```python
from build123d import *

# Parameters (mm, degrees)
SKETCH1_R           = 0.3
SKETCH1_W           = 2
SKETCH1_H           = 1.5
BOSS_EXTRUDE1_DEPTH = 1.7272


with BuildPart() as part:
    # Sketch1 → Boss-Extrude1 (new body)
    # profile 1 of 3: a face of its own
    with BuildSketch(Plane(origin=(0, 0, 0), x_dir=(0, 0, -1), z_dir=(1, 0, 0))):
        with BuildLine():
            ThreePointArc((-0.95, 14.390683939), (0, 15.340683939), (0.95, 14.390683939))
            Line((0.95, 14.390683939), (0.95, 12.490683939))
            Line((0.95, 12.490683939), (2.5, 12.490683939))
            Line((2.5, 12.490683939), (2.5, 4.605171007))
            ThreePointArc((2.5, 4.605171007), (5.185747801, 0.752076956), (3.705239533, -3.705239533))
            Line((3.705239533, -3.705239533), (2.644579362, -2.644579362))
            ThreePointArc((2.644579362, -2.644579362), (0, 3.74), (-2.644579362, -2.644579362))
            Line((-2.644579362, -2.644579362), (-3.705239533, -3.705239533))
            ThreePointArc((-3.705239533, -3.705239533), (-5.185747801, 0.752076956), (-2.5, 4.605171007))
            Line((-2.5, 4.605171007), (-2.5, 12.490683939))
            Line((-2.5, 12.490683939), (-0.95, 12.490683939))
            Line((-0.95, 12.490683939), (-0.95, 14.390683939))
        make_face()
        with Locations((0, 14.690683939)):
            Circle(SKETCH1_R, mode=Mode.SUBTRACT)
    # profile 2 of 3: a face of its own
    with BuildSketch(Plane(origin=(0, 0, 0), x_dir=(0, 0, -1), z_dir=(1, 0, 0))):
        with BuildLine():
            Line((-12.571622028, 12.490683939), (-5.24, 0))
            ThreePointArc((-5.24, 0), (-5.121580996, 1.107703977), (-4.771676297, 2.165341847))
            Line((-4.771676297, 2.165341847), (-9.951862811, 10.990683939))
            Line((-9.951862811, 10.990683939), (-2.5, 10.990683939))
            Line((-2.5, 10.990683939), (-2.5, 12.490683939))
            Line((-2.5, 12.490683939), (-12.571622028, 12.490683939))
        make_face()
    # profile 3 of 3: a face of its own
    with BuildSketch(Plane(origin=(0, 0, 0), x_dir=(0, 0, -1), z_dir=(1, 0, 0))):
        with Locations((3.5, 11.740683939)):
            Rectangle(SKETCH1_W, SKETCH1_H)
    extrude(amount=BOSS_EXTRUDE1_DEPTH)


solid = part.part
```
Geometry check sheet. Reference: the model listing, model coordinates, mm. A direction names the side the tool comes from. Coordinates: 2 decimals unless noted, no trailing zeros. Order: outer loops, then holes, each group sorted by start corner. A loop starts at its lowest first (then second) coordinate and runs counter-clockwise, first axis right, second up.
Q1. Sectioned sample at D-D on x = 0.45. Record the cut outline in (y, z), and give its area (3 significant figures).
Reply:
outline: (-3.71, -3.71) arc R5.24 ccw to (4.61, -2.5) - (10.99, -2.5) - (10.99, -4.5) - (12.49, -4.5) - (12.49, -0.95) - (14.39, -0.95) arc R0.95 ccw to (14.39, 0.95) - (12.49, 0.95) - (12.49, 12.57) - (0, 5.24) arc R5.24 ccw to (-3.71, 3.71) - (-2.64, 2.64) arc R3.74 cw (long way) to (-2.64, -2.64) - close; hole (2.17, 4.77) arc R5.24 cw to (4.61, 2.5) - (10.99, 2.5) - (10.99, 9.95) - close; hole circle Ø0.6 at (14.69, 0)
area: 108 mm2
Q2. Thickness scan on probe 1 along Y at (x, z) = (1.35, 0); probe 2 along Z at (x, y) = (1.3, 3.25); probe 3 along Z at (x, y) = (0.65, 2.75). Record the ranges inside material, lowest first.
Reply:
probe 1: y = 3.74 to 14.39, 14.99 to 15.34
probe 2: z = -4.11 to -1.85, 1.85 to 4.11, 5.41 to 7.15
probe 3: z = -4.46 to -2.53, 2.53 to 4.46, 5.11 to 6.85
Q3. Sectioned sample at A-A on z = 0. Record the cut outline in (x, y), and give its area (3 significant figures).
Reply:
outline: (0, 3.74) - (1.73, 3.74) - (1.73, 14.39) - (0, 14.39) - close; (0, 14.99) - (1.73, 14.99) - (1.73, 15.34) - (0, 15.34) - close
area: 19.0 mm2
Q4. Draft check along Y on faces 4 (the face through (0.852, 6.333, 8.957)), 5 (the face through (0.852, 0.819, -5.176)), 6 (the face through (1, 12.491, -3)), 7 (the face through (0.852, 3.553, 3.851)). Enter one of: released by +Y, released by -Y, zero draft, split by the parting line, or undercut.
Reply:
face 4: released by -Y
face 5: undercut
face 6: released by +Y
face 7: undercut
Q5. Sectioned sample at B-B on y = 3. Record the cut outline in (x, z), and give its area (3 significant figures).
Reply:
outline: (0, -4.3) - (1.73, -4.3) - (1.73, -2.23) - (0, -2.23) - close; (0, 2.23) - (1.73, 2.23) - (1.73, 4.3) - (0, 4.3) - close; (0, 5.26) - (1.73, 5.26) - (1.73, 7) - (0, 7) - close
area: 10.1 mm2
Q6. Tool access check on faces 1 (the face through (1, 13, -0.95)), 2 (the face through (1, 12.491, 7)), 3 (the face through (1, 8, 2.5)). Record the directions out of +Z, -Z, +X, -X, +Y, -Y that give a thin tool (end or side, any length) a straight path to the whole face; none if there is none.
Reply:
face 1: -Z, +X, -X, +Y
face 2: +Z, +X, -X, +Y
face 3: +X, -X
Q7. Depth check by flat-ended pin: pin 1 Ø0.5 at (x, z) = (1, -3) entering from -Y; pin 2 Ø1 at (x, y) = (1.5, 6.5) entering from -Z; pin 3 Ø6.5 at (y, z) = (0, 0) entering from -X; pin 4 Ø0.9 at (x, y) = (1, 9) entering from +Z. Enter the tip coordinate at first touch or a pass-through.
Reply:
pin 1: stops at y = -3.25
pin 2: stops at z = -2.5
pin 3: passes through
pin 4: stops at z = 10.79
Q8. Sectioned sample at C-C on y = 7.25. Record the cut outline in (x, z), and give its area (3 significant figures).
Reply:
outline: (0, -2.5) - (1.73, -2.5) - (1.73, 2.5) - (0, 2.5) - close; (0, 7.76) - (1.73, 7.76) - (1.73, 9.5) - (0, 9.5) - close
area: 11.6 mm2
